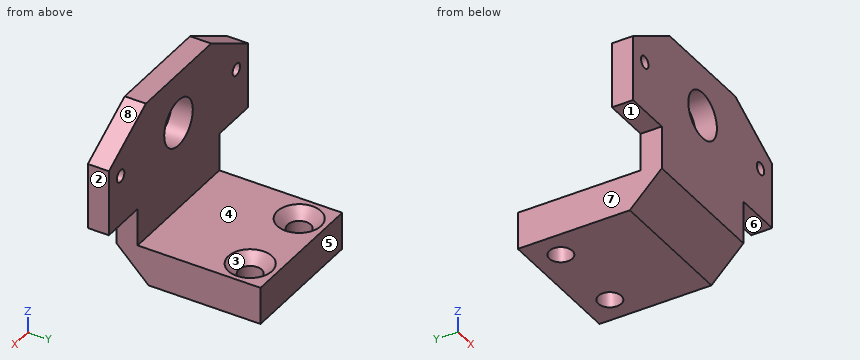
from build123d import *

# Parameters (mm, degrees)
BOSS_EXTRUDE1_DEPTH                             = 5.0292
SKETCH2_W                                       = 31.75
SKETCH2_H                                       = 8.89
BOSS_EXTRUDE2_DEPTH                             = 34.29
CUT_EXTRUDE1_DEPTH                              = 61.675621628
CUT_EXTRUDE1_DEPTH_BACK                         = 61.675621628
CSK_FOR_M5_FLAT_HEAD_MACHINE_SCREW1_D           = 5.5
CSK_FOR_M5_FLAT_HEAD_MACHINE_SCREW1_CSINK_D     = 10.4
CSK_FOR_M5_FLAT_HEAD_MACHINE_SCREW1_CSINK_ANGLE = 90
SKETCH7_R                                       = 5.55625
CUT_EXTRUDE2_DEPTH                              = 48.445089331
M2_5_CLEARANCE_HOLE1_D                          = 2.9


with BuildPart() as part:
    # Sketch1 → Boss-Extrude1 (new body)
    with BuildSketch(Plane(origin=(0, 0, 0), x_dir=(1, 0, 0), z_dir=(0, 1, 0))):
        Polygon((-27.051, 7.874), (-15.875, 7.874), (-15.875, 16.860446287), (15.875, 16.860446287), (15.875, 7.874), (27.051, 7.874), (27.051, -7.874), (12.7, -16.159553713), (-12.7, -16.159553713), (-27.051, -7.874), align=None)
    extrude(amount=BOSS_EXTRUDE1_DEPTH)

    # Sketch2 → Boss-Extrude2 (add)
    with BuildSketch(Plane(origin=(0, 0, 0), x_dir=(1, 0, 0), z_dir=(0, 1, 0))):
        with Locations((0, 21.305446287)):
            Rectangle(SKETCH2_W, SKETCH2_H)
    extrude(amount=BOSS_EXTRUDE2_DEPTH)

    # Sketch3 → Cut-Extrude1 (cut, two sides: drawn at the far end of the back side and taken through both)
    with BuildSketch(Plane(origin=(15.875, 0, 0), x_dir=(0, 0, -1), z_dir=(1, 0, 0)).offset(-CUT_EXTRUDE1_DEPTH_BACK)):
        Polygon((103.074442863, 84.943996576), (25.750446287, 7.62), (18.130446287, 0), (-59.19355029, -77.323996576), (95.454442863, -231.971989729), (257.722436016, -69.703996576), align=None)
    extrude(amount=CUT_EXTRUDE1_DEPTH + CUT_EXTRUDE1_DEPTH_BACK, mode=Mode.SUBTRACT)

    # CSK for M5 Flat Head Machine Screw1 (through all)
    with Locations(Plane.XY.offset(-16.860446287)):
        with Locations((-9.525, 27.94), (9.525, 27.94)):
            CounterSinkHole(CSK_FOR_M5_FLAT_HEAD_MACHINE_SCREW1_D / 2, CSK_FOR_M5_FLAT_HEAD_MACHINE_SCREW1_CSINK_D / 2, counter_sink_angle=CSK_FOR_M5_FLAT_HEAD_MACHINE_SCREW1_CSINK_ANGLE)

    # Sketch7 → Cut-Extrude2 (cut, through all)
    with BuildSketch(Plane(origin=(0, 5.0292, 0), x_dir=(1, 0, 0), z_dir=(0, 1, 0))):
        with Locations(Location((0, -4.064, 0), (0, 0, 270))):
            Circle(SKETCH7_R)
    extrude(amount=-CUT_EXTRUDE2_DEPTH, mode=Mode.SUBTRACT)

    # M2.5 Clearance Hole1 (through all)
    with Locations(Plane(origin=(0, 5.0292, 0), x_dir=(1, 0, 0), z_dir=(0, 1, 0))):
        with Locations((-22.5, -4.064), (22.5, -4.064)):
            Hole(M2_5_CLEARANCE_HOLE1_D / 2)


solid = part.part
The model under review builds one solid part; all positions refer to its coordinate system, in mm. Face numbers are marked on the shaded views. A direction names the side the tool comes from. Coordinates: 2 decimals unless noted, no trailing zeros. Order: outer loops, then holes, each group sorted by start corner. A loop starts at its lowest first (then second) coordinate and runs counter-clockwise, first axis right, second up. Notation, with made-up numbers: (-29.75, -6) -> (16.25, -6) arc R24 ccw to (16.25, 13) -> close; hole circle Ø3 at (26.5, 19.5). An arc over 180 degrees is marked (long way). Answer in a Markdown table with one row per item.
(1) Consider section B-B (y = 27.94). Write out the cut boundary in (x, z) (3 decimals), plus the area to 3 significant figures.
Answers:
| item | result |
|---|---|
| outline | (-15.875, -25.75) -> (-12.275, -25.75) -> (-12.275, -19.31) -> (-14.725, -16.86) -> (-15.875, -16.86) -> close; (-6.775, -25.75) -> (6.775, -25.75) -> (6.775, -19.31) -> (4.325, -16.86) -> (-4.325, -16.86) -> (-6.775, -19.31) -> close; (12.275, -25.75) -> (15.875, -25.75) -> (15.875, -16.86) -> (14.725, -16.86) -> (12.275, -19.31) -> close |
| area | 172 mm² |
(2) Wall thickness on line 1 along X through (y, z) = (27.94, -24.25) (3 decimals); line 2 along Y through (x, z) = (-3.5, -13.5); line 3 along X through (y, z) = (12, -24) (3 decimals): over which ranges is each line inside the solid? List them lowest first.
Answers:
| item | result |
|---|---|
| line 1 | -15.875 to -12.275, -6.775 to 6.775, 12.275 to 15.875 |
| line 2 | 0 to 5.03 |
| line 3 | -15.875 to 15.875 |
(3) Insertion check: pin 1 (16.5 mm diameter, centred on x = -13, z = -8, fed in from +Y); pin 2 (14.5 mm diameter, centred on y = 24.5, z = -17.5, fed in from -X) (3 decimals); pin 3 (1.5 mm diameter, centred on x = 24, y = 3.5, fed in from -Z); pin 4 (3.5 mm diameter, centred on x = 9.525, y = 27.94, fed in from +Z). Each pin has a flat end and moves straight along its axis. Give the tip position at first contact, or say it passes through.
Answers:
| item | result |
|---|---|
| pin 1 | y = 5.03 |
| pin 2 | x = -15.875 |
| pin 3 | z = -7.87 |
| pin 4 | through |
(4) Consider section C-C (z = 0). Write out the cut boundary in (x, y).
Answers:
| item | result |
|---|---|
| outline | (-27.05, 0) -> (-3.79, 0) -> (-3.79, 5.03) -> (-27.05, 5.03) -> close; (3.79, 0) -> (27.05, 0) -> (27.05, 5.03) -> (3.79, 5.03) -> close |
(5) Machinability: for the marked faces 4, 5, 6, 7 and 8, which of the approach directions +Z, -Z, +X, -X, +Y, -Y give a long, thin tool a straight path to every point of the face, cutting with its end or side? Answer none if there is none.
Answers:
| item | result |
|---|---|
| face 4 | +Z, +X, -X, +Y |
| face 5 | +Z, -Z, +X, -X, +Y |
| face 6 | -Z, +X, +Y, -Y |
| face 7 | -Z, -X, +Y, -Y |
| face 8 | +Z, +X, +Y, -Y |
(6) Consider section D-D (z = -5). Write out the cut boundary in (x, y).
Answers:
| item | result |
|---|---|
| outline | (-27.05, 0) -> (27.05, 0) -> (27.05, 5.03) -> (-27.05, 5.03) -> close |
(7) Consider section A-A (x = 0). Write out the cut boundary in (y, z).
Answers:
| item | result |
|---|---|
| outline | (0, -18.13) -> (7.62, -25.75) -> (34.29, -25.75) -> (34.29, -16.86) -> (5.03, -16.86) -> (5.03, -1.49) -> (0, -1.49) -> close; (0, 9.62) -> (5.03, 9.62) -> (5.03, 16.16) -> (0, 16.16) -> close |
(8) The part is to be moulded in two halves that separate along X. For the marked faces 1, 2 and 3, say which applies: +X half, -X half, draft (parallel to the pull), parting line (faces both ways), or undercut.
Answers:
| item | result |
|---|---|
| face 1 | draft |
| face 2 | +X half |
| face 3 | undercut |
